The listing builds one solid part. Answer for the finished solid, in the listing's coordinates (mm). Face numbers are marked on the shaded views. A direction names the side the tool comes from. Round coordinates to 2 decimals unless told otherwise and drop trailing zeros. Loops run counter-clockwise (first coordinate to the right, second up) from the corner with the lowest first, then second, coordinate; pieces in that order, holes last. Notation, with made-up numbers: M 58.25,-12 L 114.25,-12 A19 ccw 114.25,19 Z; hole C 49,-17.5 d10. An arc over 180 degrees is marked long. Answer as a JSON object with one key per item and string values.
Autodesk Inventor part; units mm, degrees
ref_plane "YZ Plane" through (0, 0, 0) normal (1, 0, 0) x (0, 1, 0)
ref_plane "XZ Plane" through (0, 0, 0) normal (0, 1, 0) x (-1, 0, 0)
ref_plane "XY Plane" through (0, 0, 0) normal (0, 0, 1) x (1, 0, 0)
sketch "Sketch1" plane through (0, 0, 0) normal (0, 1, 0) x (-1, 0, 0)
  line L0 (0.85, 3.2) -> (-0.85, 3.2)
  line L1 (-0.85, 3.2) -> (-0.85, -3.2)
  line L2 (-0.85, -3.2) -> (0.85, -3.2)
  line L3 (0.85, -3.2) -> (0.85, 3.2)
  line L4 (0.85, 3.2) -> (-0.85, -3.2) construction
  line L5 (-0.85, 3.2) -> (0.85, -3.2) construction
  line L6 (-0.85, -1.3) -> (-2.35, -1.3) construction
  line L7 (-2.35, -1.3) -> (-2.35, -3.4525)
  line L8 (-0.85, -3.2) -> (-0.85, -1.3)
  line L9 (-2.35, -3.4525) -> (-2.35, -3.8)
  line L10 (-2.35, -3.8) -> (-0.85, -3.8)
  line L11 (-0.85, -3.8) -> (-0.85, -3.2)
  line L12 (-2.35, -2.5) -> (-0.85, -2.5)
  line L13 (0, 0) -> (-4.1965, 0) construction
  line L14 (-2.35, 1.3) -> (-2.35, 3.4525)
  line L15 (-2.35, 2.5) -> (-0.85, 2.5)
  line L16 (-0.85, 2.5) -> (-2.35, 2.5)
  line L17 (-2.35, 2.5) -> (-2.35, 4.2)
  line L18 (-2.35, 4.2) -> (-0.85, 4.2)
  line L19 (-0.85, 4.2) -> (-0.85, 2.5)
  line L20 (-0.85, 2.5) -> (-0.15, 2.5)
  line L21 (-0.15, 2.5) -> (-0.15, -2.5)
  line L22 (-0.15, -2.5) -> (-0.85, -2.5)
  line L23 (-0.85, -2.5) -> (-0.85, 2.5)
  point P0 (-0.85, 2.5)
  point P1 (-0.85, -2.5)
  point P2 (-2.35, 3.4525)
  dimension "d0" = 1.3
  dimension "d2" = 1.7
  dimension "d3" = 1.5
  dimension "d5" = 1.9
  dimension "d7" = 2.5
  dimension "d13" = 1
  dimension "d14" = 2.5
  dimension "d18" = 0.7
extrude "Extrusion1" add sketch "Sketch1" along normal blind 2.8 contours L3 L2 L1 L22 L21 L20 L0 | L1 L15 L14 L17 L18 L19 | L11 L10 L9 L7 L12 L1
sketch "Sketch2" plane through (0, 0, 0) normal (0, 0, 1) x (1, 0, 0)
  line L0 (0.85, 2.8) -> (2.35, 2.8)
  line L1 (2.35, 2.8) -> (2.35, 1.3)
  line L2 (2.35, 1.3) -> (0.85, 1.3)
  line L3 (0.85, 1.3) -> (0.85, 2.8)
  line L4 (2.35, 0) -> (2.35, 2.8)
  line L5 (0.85, 0) -> (0.85, 2.8)
  line L6 (0.85, 2.8) -> (2.35, 2.8)
  dimension "d15" = 1.5
extrude "Extrusion2" cut sketch "Sketch2" along normal through all both and the other way through all
fillet "Fillet1" radius 0.8 2 edges at (0.15, 1.4, -2.5) (0.15, 1.4, 2.5)
fillet "Fillet1" radius 1 2 edges at (0.85, 1.3, 2.85) (0.85, 1.3, -2.85)
fillet "Fillet1" radius 0.4 2 edges at (2.35, 1.3, 3.35) (2.35, 1.3, -3.15)
fillet "Fillet1" radius 0.4 4 edges at (-0.85, 2.8, 0) (-0.85, 0, 0) (-0.85, 1.4, -3.2) (-0.85, 1.4, 3.2)
equation "\"button_height\" = 1.3"
properties part number "Button"
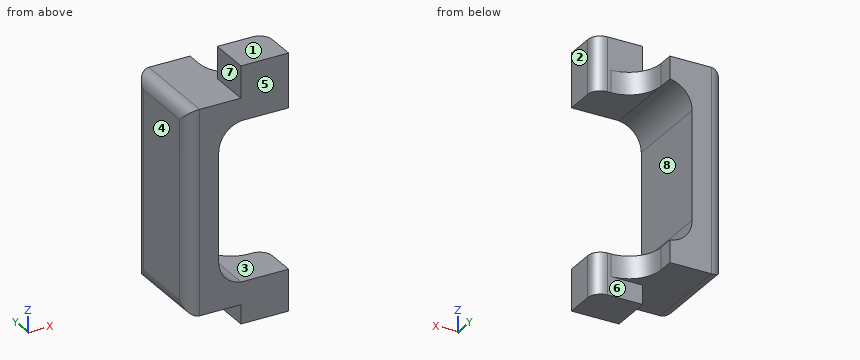
Item 1: The part is cut by section A-A (x = 1.05). Give the vertices of the cut face in (y, z), then the cut area to 3 significant figures.
Values follow:
{"outline": "M 0,-3.8 L 1.3,-3.8 L 1.3,-3.2 L 1.7,-3.2 L 1.7,-2.5 L 0,-2.5 Z; M 0,2.5 L 1.7,2.5 L 1.7,3.2 L 1.3,3.2 L 1.3,4.2 L 0,4.2 Z", "area": "4.46 mm^2"}
Item 2: Flat-ended cylindrical pins translate along their axes: P1, Ø0.8, axis at y = 1, z = 4, coming from the -X side; P2, Ø1.5, axis at x = 0, y = 0.5, coming from the -Z side; P3, Ø1.4, axis at y = 1, z = -0.5, coming from the +X side; P4, Ø0.8, axis at x = 1.5, y = 1.5, coming from the -Z side. Find the tip coordinate at first contact, or state that the pin passes through.
Values follow:
{"P1": "x = 0.85", "P2": "z = -3.2", "P3": "x = 0.15", "P4": "z = -3.8"}
Item 3: Which of the six approach directions +Z, -Z, +X, -X, +Y, -Y give full straight-line access (tool end or side, diameter ignored) to the marked faces 4, 5, 6, 7 and 8?
Values follow:
{"face 4": "+Z, -Z, -X, +Y, -Y", "face 5": "+Z, -Z, +X, -X, -Y", "face 6": "-Z, +X, +Y", "face 7": "+Z, -X, +Y, -Y", "face 8": "+X, +Y, -Y"}
Item 4: Determine the mould class of the marked faces 1, 2 and 3 for opening direction Z: released by +Z, released by -Z, zero draft, split by the parting line, or undercut.
Values follow:
{"face 1": "released by +Z", "face 2": "zero draft", "face 3": "undercut"}
Item 5: Straight lines are drawn through the part: line 1 (Z direction, x = 0.9, y = 0.7); line 2 (Y direction, x = 1.55, z = 3.25); line 3 (Z direction, x = 0.4, y = 0.4). For each, find the intervals that lie inside material, in ascending order.
Values follow:
{"line 1": "-3.8 to -2.5, 2.5 to 4.2", "line 2": "0 to 1.3", "line 3": "-3.2 to -2.28, 2.28 to 3.2"}
Item 6: The part is cut by section C-C (z = 1.5). Give the vertices of the cut face in (x, y), then the cut area to 3 significant figures.
Values follow:
{"outline": "M -0.85,0.4 A0.4 ccw -0.45,0 L 0.15,0 L 0.15,2.8 L -0.45,2.8 A0.4 ccw -0.85,2.4 Z", "area": "2.73 mm^2"}
